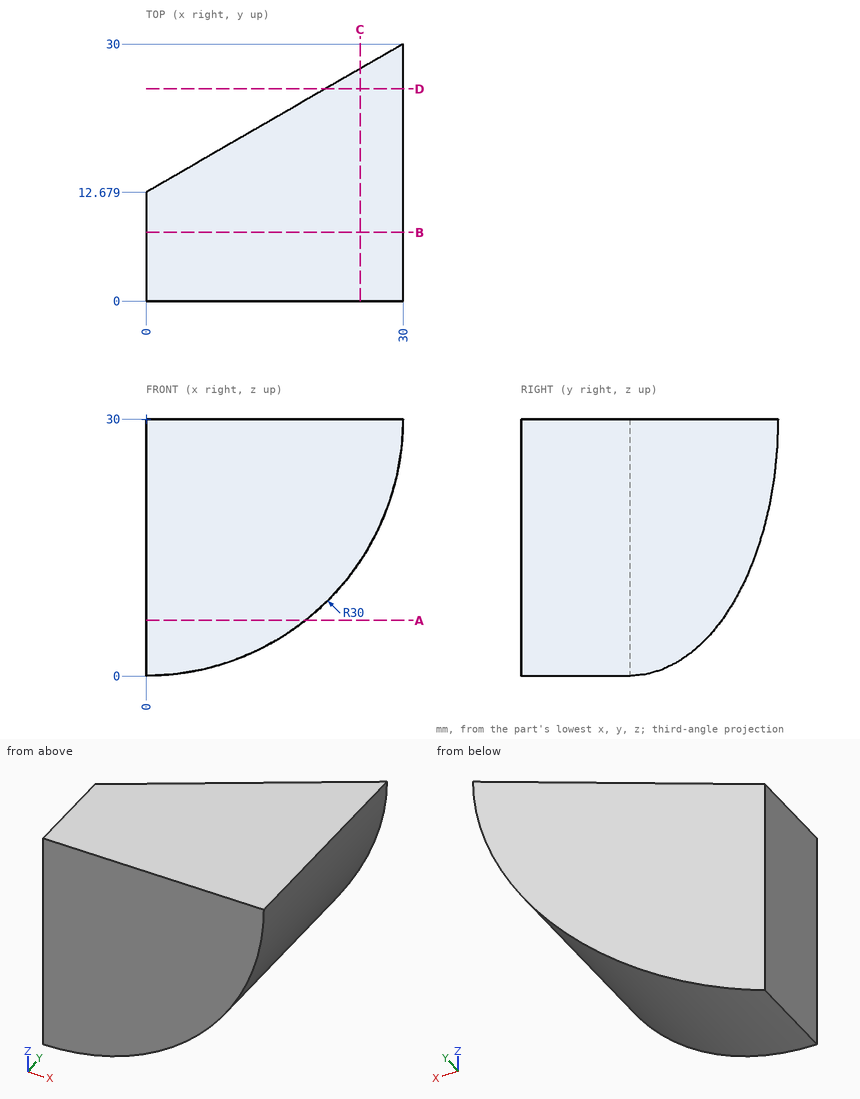
Part print with two shaded views. Sizes in mm from the minimum x, y, z corner. Round coordinates to 2 decimals unless told otherwise and drop trailing zeros. Order: outer loops, then holes, each group sorted by start corner. A loop starts at its lowest first (then second) coordinate and runs counter-clockwise, first axis right, second up. Notation, with made-up numbers: M 59,59.5 L 92,59.5 A32 cw 92,90.5 Z; hole C 78,62.5 d8. An arc over 180 degrees is marked long. Put each result on its own line as item: value. Start each with the question number.
1. Slice it at C-C on x = 25. List the corners of the cut face in (y, z).
2. Slice it at B-B on y = 8. List the corners of the cut face in (x, z).
3. Drop flat-ended pins along their axis: pin 1 (10 mm diameter, centred on y = 5.5, z = 15.5, fed in from +X); pin 2 (6 mm diameter, centred on x = 11.5, z = 4.5, fed in from +Y); pin 3 (10 mm diameter, centred on x = 7, y = 19.5, fed in from -Z) (1 decimal). Give the stop position or say it passes through.
4. Drill centre lines: probe 1 along Z at (x, y) = (20.5, 15.75) (1 decimal); probe 2 along Y at (x, z) = (6.25, 17); probe 3 along X at (y, z) = (20, 21) (1 decimal). Where is each one in solid material? Low to high. Write a range as [from, to].
5. Slice it at D-D on y = 24.75. List the corners of the cut face in (x, z) (1 decimal).
6. Slice it at A-A on z = 6.5. List the corners of the cut face in (x, y) (1 decimal), then the cut area to 3 significant figures.
Findings:
1. outline: M 0,13.42 L 27.11,13.42 L 27.11,30 L 0,30 Z
2. outline: M 0,0 A30 ccw 30,30 L 0,30 Z
3. pin 1: x = 28.46
3. pin 2: y = 21.05
3. pin 3: z = 0.3
4. probe 1: [8.1, 30]
4. probe 2: [0, 16.29]
4. probe 3: [12.7, 28.6]
5. outline: M 20.9,8.5 A30 ccw 30,30 L 20.9,30 Z
6. outline: M 0,0 L 18.6,0 L 18.6,23.4 L 0,12.7 Z
6. area: 337 mm2
